from build123d import *

# Parameters (mm, degrees)
SKETCH2_W             = 40
SKETCH2_H             = 20
BOSS_EXTRUDE1_DEPTH   = 27.65
SKETCH3_W             = 7
SKETCH3_H             = 4
BOSS_EXTRUDE2_DEPTH   = 5
SKETCH5_W             = 40
SKETCH5_H             = 20
BOSS_EXTRUDE5_DEPTH   = 12.8
SKETCH7_W             = 20
SKETCH7_H             = 4
BOSS_EXTRUDE6_DEPTH   = 7.22
CUT_EXTRUDE3_DEPTH    = 4
MIRROR11_COPY_1_DEPTH = 4
SKETCH9_R             = 6.5
BOSS_EXTRUDE8_DEPTH   = 1.5


with BuildPart() as part:
    # Sketch2 → Boss-Extrude1 (new body)
    with BuildSketch(Plane(origin=(0, 0, 0), x_dir=(1, 0, 0), z_dir=(0, 1, 0))):
        Rectangle(SKETCH2_W, SKETCH2_H)
    extrude(amount=BOSS_EXTRUDE1_DEPTH)

    # Sketch3 → Boss-Extrude2 (add)
    with BuildSketch(Plane.ZY.offset(20)):
        with Locations((0, 6)):
            Rectangle(SKETCH3_W, SKETCH3_H)
    extrude(amount=BOSS_EXTRUDE2_DEPTH)

    # Sketch5 → Boss-Extrude5 (add)
    with BuildSketch(Plane(origin=(0, 27.65, 0), x_dir=(1, 0, 0), z_dir=(0, 1, 0))):
        Rectangle(SKETCH5_W, SKETCH5_H)
    extrude(amount=BOSS_EXTRUDE5_DEPTH)

    # Sketch7 → Boss-Extrude6 (add)
    with BuildSketch(Plane.ZY.offset(20)):
        with Locations((0, 29.65)):
            Rectangle(SKETCH7_W, SKETCH7_H)
    boss_extrude6 = extrude(amount=BOSS_EXTRUDE6_DEPTH)

    # Sketch8 → Cut-Extrude3 (cut)
    with BuildSketch(Plane(origin=(0, 31.65, 0), x_dir=(1, 0, 0), z_dir=(0, 1, 0))):
        with BuildLine():
            Line((-26.265564437, 6), (-27.22, 6))
            Line((-27.22, 6), (-27.22, 4))
            Line((-27.22, 4), (-26.265564437, 4))
            ThreePointArc((-26.265564437, 4), (-22, 5), (-26.265564437, 6))
        make_face()
    cut_extrude3 = extrude(amount=-CUT_EXTRUDE3_DEPTH, mode=Mode.SUBTRACT)

    # Mirror10: Cut-Extrude3 across plane
    add(cut_extrude3.mirror(Plane.XY), mode=Mode.SUBTRACT)

    # Mirror11: Boss-Extrude6, Cut-Extrude3 across plane
    add(boss_extrude6.mirror(Plane(origin=(0, 0, 0), x_dir=(0, 0, 1), z_dir=(1, 0, 0))))
    add(cut_extrude3.mirror(Plane(origin=(0, 0, 0), x_dir=(0, 0, 1), z_dir=(1, 0, 0))), mode=Mode.SUBTRACT)

    # Mirror11 copy 1 sketch → Mirror11 copy 1 (cut)
    with BuildSketch(Plane(origin=(0, 31.65, 0), x_dir=(-1, 0, 0), z_dir=(0, 1, 0))):
        with BuildLine():
            Line((-26.265564437, 6), (-27.22, 6))
            Line((-27.22, 6), (-27.22, 4))
            Line((-27.22, 4), (-26.265564437, 4))
            ThreePointArc((-26.265564437, 4), (-22, 5), (-26.265564437, 6))
        make_face()
    extrude(amount=-MIRROR11_COPY_1_DEPTH, mode=Mode.SUBTRACT)

    # Sketch9 → Boss-Extrude8 (add)
    with BuildSketch(Plane(origin=(0, 40.45, 0), x_dir=(1, 0, 0), z_dir=(0, 1, 0))):
        with Locations(Location((-9.95, 0, 0), (0, 0, 270))):
            Circle(SKETCH9_R)
    extrude(amount=BOSS_EXTRUDE8_DEPTH)


solid = part.part
Read the model definition and answer for the solid it produces. Units are mm, in the model's axes. A direction names the side the tool comes from. Coordinates: 2 decimals unless noted, no trailing zeros. Loops run counter-clockwise (first coordinate to the right, second up) from the corner with the lowest first, then second, coordinate; pieces in that order, holes last. Notation, with made-up numbers: (61.5, -22) -> (100.5, -22) arc R19 ccw to (100.5, -8) -> close; hole circle Ø1 at (42, 74). An arc over 180 degrees is marked (long way). Answer in a Markdown table with one row per item.
Item 1: A cutting plane is placed at C-C on x = -5. Determine the outline of the cut face in (y, z), plus the area to 3 significant figures.
Returned:
| item | result |
|---|---|
| outline | (0, -10) -> (40.45, -10) -> (40.45, -4.21) -> (41.95, -4.21) -> (41.95, 4.21) -> (40.45, 4.21) -> (40.45, 10) -> (0, 10) -> close |
| area | 822 mm^2 |
Item 2: For a pull along Y with two mould halves and no side action, classify faces 1 (the flat face through (27.22, 30, 8)), 2 (the flat face through (-20, 14, 0)), 3 (the flat face through (-10, 41.95, 0)) as released by +Y, released by -Y, zero draft, split by the parting line, or undercut.
Returned:
| item | result |
|---|---|
| face 1 | zero draft |
| face 2 | undercut |
| face 3 | released by +Y |
Item 3: A cutting plane is placed at B-B on z = 0. Determine the outline of the cut face in (x, y), plus the area to 3 significant figures.
Returned:
| item | result |
|---|---|
| outline | (-27.22, 27.65) -> (-20, 27.65) -> (-20, 8) -> (-25, 8) -> (-25, 4) -> (-20, 4) -> (-20, 0) -> (20, 0) -> (20, 27.65) -> (27.22, 27.65) -> (27.22, 31.65) -> (20, 31.65) -> (20, 40.45) -> (-3.45, 40.45) -> (-3.45, 41.95) -> (-16.45, 41.95) -> (-16.45, 40.45) -> (-20, 40.45) -> (-20, 31.65) -> (-27.22, 31.65) -> close |
| area | 1,720 mm^2 |
Item 4: For faces 4 (the cylindrical face through (-22, 30, -5)), 5 (the flat face through (-22, 8, 0)), 6 (the flat face through (-22, 4, 0)), 7 (the flat face through (20, 14, 0)), 8 (the flat face through (20, 36, 0)), determine the directions among +Z, -Z, +X, -X, +Y, -Y from which every point of the face is accessible in a straight line to the end or side of a thin tool.
Returned:
| item | result |
|---|---|
| face 4 | +Y |
| face 5 | +Z, -Z, -X |
| face 6 | +Z, -Z, -X, -Y |
| face 7 | +Z, -Z, +X, -Y |
| face 8 | +Z, -Z, +X, +Y |
Item 5: Straight lines are drawn through the part: line 1 along Z through (x, y) = (-24.25, 28.65); line 2 along Y through (x, z) = (-15.5, -6.25); line 3 along X through (y, z) = (29.25, 5). For each, find the intervals that lie inside material, in ascending order. Write a range as [from, to].
Returned:
| item | result |
|---|---|
| line 1 | z = [-10, -7.25], [-2.75, 2.75], [7.25, 10] |
| line 2 | y = [0, 40.45] |
| line 3 | x = [-22, 22] |
Item 6: Each of these flat-tipped pins is pushed along its axis until it touches: P1, Ø2, axis at x = 22, z = 4.5, coming from the -Y side; P2, Ø5, axis at x = -15.5, z = -7, coming from the +Y side; P3, Ø10, axis at y = 14, z = -3, coming from the +X side; P4, Ø5.5, axis at x = -22, z = 0.5, coming from the +Y side. Where does it stop, or does it pass through?
Returned:
| item | result |
|---|---|
| P1 | stops at y = 27.65 |
| P2 | stops at y = 41.95 |
| P3 | stops at x = 20 |
| P4 | stops at y = 40.45 |
Item 7: A cutting plane is placed at D-D on y = 36.5. Determine the outline of the cut face in (x, z).
Returned:
| item | result |
|---|---|
| outline | (-20, -10) -> (20, -10) -> (20, 10) -> (-20, 10) -> close |
Item 8: A cutting plane is placed at A-A on x = -24.25. Determine the outline of the cut face in (y, z).
Returned:
| item | result |
|---|---|
| outline | (4, -3.5) -> (8, -3.5) -> (8, 3.5) -> (4, 3.5) -> close; (27.65, -10) -> (31.65, -10) -> (31.65, -7.25) -> (27.65, -7.25) -> close; (27.65, -2.75) -> (31.65, -2.75) -> (31.65, 2.75) -> (27.65, 2.75) -> close; (27.65, 7.25) -> (31.65, 7.25) -> (31.65, 10) -> (27.65, 10) -> close |
